Answer from the drawing. Dimensions are ordinates in mm from the lowest x, y and z of the part. Give positions to 0.01 mm unless a question says otherwise; leave off trailing zeros. Write each loop counter-clockwise with the first axis right and the second up, starting at its lowest first coordinate (ties: lowest second). Pieces come first, ordered by that corner, then holes. Notation, with made-up numbers: M -0.75,9 L 50.25,9 A13 ccw 50.25,16 Z; hole C -37,-15.5 d2. An arc over 180 degrees is marked long. Answer as a JSON object with one key per item and string values.
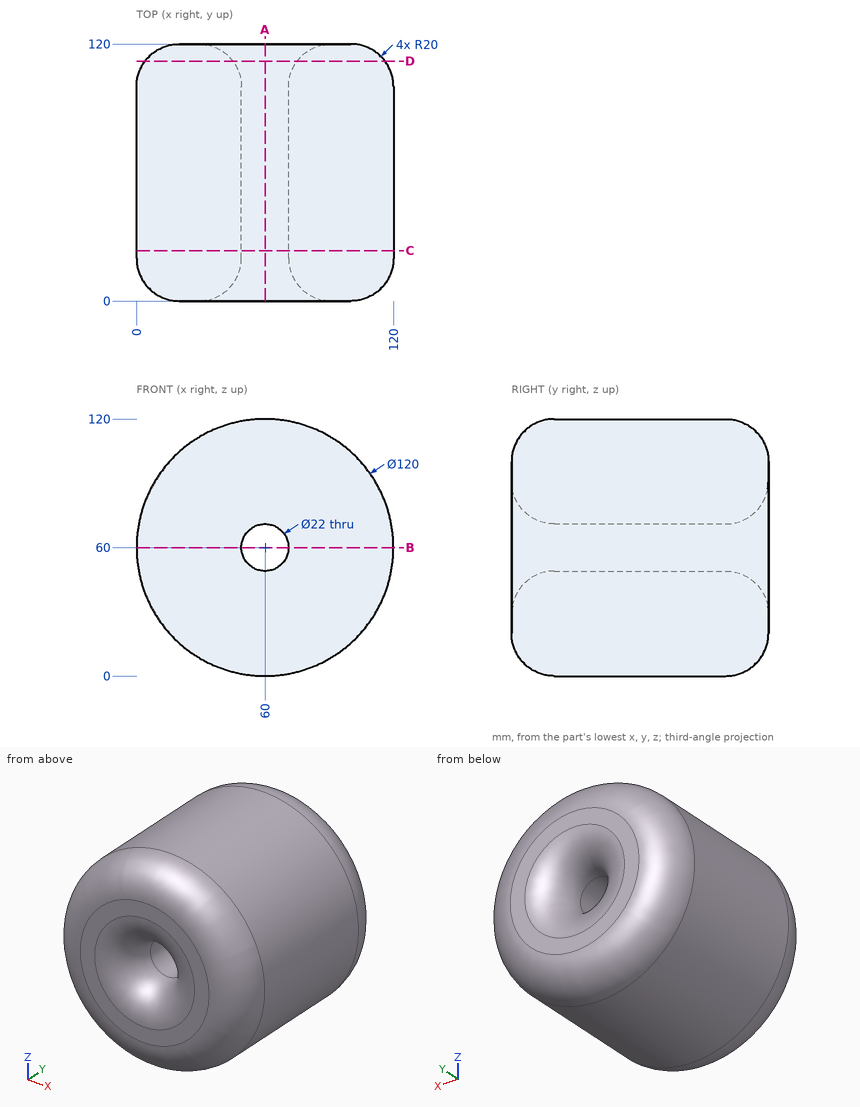
1. A cutting plane is placed at A-A, the plane x = 60. Give the vertices of the cut face in (y, z).
Verdict:
{"outline": "M 0,20 A20 ccw 20,0 L 100,0 A20 ccw 120,20 L 120,29 A20 ccw 100,49 L 20,49 A20 ccw 0,29 Z; M 0,91 A20 ccw 20,71 L 100,71 A20 ccw 120,91 L 120,100 A20 ccw 100,120 L 20,120 A20 ccw 0,100 Z"}
2. Consider line 1 along Z through (x, y) = (60, 56); line 2 along Z through (x, y) = (54.5, 10.5); line 3 along X through (y, z) = (26, 65.5). Determine where each line is inside the solid, lowest interval first.
Verdict:
{"line 1": "z = 0 to 49, 71 to 120", "line 2": "z = 2.66 to 47.78, 72.22 to 117.34", "line 3": "x = 0.25 to 50.47, 69.53 to 119.75"}
3. Flat-ended cylindrical pins translate along their axes: pin 1 (1 mm diameter, centred on y = 76.5, z = 19.5, fed in from +X); pin 2 (3 mm diameter, centred on x = 35, z = 59.5, fed in from +Y); pin 3 (5 mm diameter, centred on y = 29.5, z = 15.5, fed in from -X). Find the tip coordinate at first contact, or state that the pin passes through.
Verdict:
{"pin 1": "stops at x = 104.72", "pin 2": "stops at y = 119.49", "pin 3": "stops at x = 17.15"}
4. A cutting plane is placed at C-C, the plane y = 23.5. Give the vertices of the cut face in (x, z).
Verdict:
{"outline": "C 60,60 d120; hole C 60,60 d22"}
5. A cutting plane is placed at B-B, the plane z = 60. Give the vertices of the cut face in (x, y), plus the area to 3 significant figures.
Verdict:
{"outline": "M 0,20 A20 ccw 20,0 L 29,0 A20 ccw 49,20 L 49,100 A20 ccw 29,120 L 20,120 A20 ccw 0,100 Z; M 71,20 A20 ccw 91,0 L 100,0 A20 ccw 120,20 L 120,100 A20 ccw 100,120 L 91,120 A20 ccw 71,100 Z", "area": "11,100 mm2"}
6. A cutting plane is placed at D-D, the plane y = 112. Give the vertices of the cut face in (x, z).
Verdict:
{"outline": "C 60,60 d112; hole C 60,60 d30"}
